```python
from build123d import *

# Parameters (mm, degrees)
SKETCH010_W     = 150
SKETCH010_H     = 108.5
PAD004_DEPTH    = 3
SKETCH011_W     = 3
SKETCH011_H     = 108.5
PAD005_DEPTH    = 36.8
SKETCH014_R     = 1.7
POCKET006_DEPTH = 5
SKETCH015_R     = 1.7
POCKET007_DEPTH = 5
POCKET010_DEPTH = 5
FILLET_R        = 2


with BuildPart() as part:
    # Sketch010 → Pad004 (new body)
    with BuildSketch(Plane.XY):
        with Locations((100.092897, -83.705943)):
            Rectangle(SKETCH010_W, SKETCH010_H)
    extrude(amount=PAD004_DEPTH)

    # Sketch011 (on Face5 of Pad004) → Pad005 (join)
    with BuildSketch(Plane(origin=(0, 0, 0), x_dir=(1, 0, 0), z_dir=(0, 0, -1))):
        with Locations((173.592904, 83.705948)):
            Rectangle(SKETCH011_W, SKETCH011_H)
        with Locations((26.592904, 83.705948)):
            Rectangle(SKETCH011_W, SKETCH011_H)
    extrude(amount=PAD005_DEPTH)

    # Sketch014 (on Face15 of Pad005) → Pocket006 (cut)
    with BuildSketch(Plane.YZ.offset(175.092904)):
        with Locations((-134.353821, -32.656531)):
            Circle(SKETCH014_R)
        with Locations((-33.353821, -32.656531)):
            Circle(SKETCH014_R)
    extrude(amount=-POCKET006_DEPTH, mode=Mode.SUBTRACT)

    # Sketch015 (on Face13 of Pocket006) → Pocket007 (cut)
    with BuildSketch(Plane(origin=(25.092904, 0, 0), x_dir=(0, -1, 0), z_dir=(-1, 0, 0))):
        with Locations((33.054447, -32.772871)):
            Circle(SKETCH015_R)
        with Locations((134.054447, -32.772871)):
            Circle(SKETCH015_R)
    extrude(amount=-POCKET007_DEPTH, mode=Mode.SUBTRACT)

    # Sketch018 (on Face13 of Pocket007) → Pocket010 (cut)
    with BuildSketch(Plane(origin=(25.092904, 0, 0), x_dir=(0, -1, 0), z_dir=(-1, 0, 0))):
        with BuildLine():
            ThreePointArc((48.372218, -10.337513), (46.972218, -8.937513), (45.572218, -10.337513))
            Line((45.572218, -10.337513), (45.572218, -26.337513))
            ThreePointArc((45.572218, -26.337513), (46.972218, -27.737513), (48.372218, -26.337513))
            Line((48.372218, -10.337513), (48.372218, -26.337513))
        make_face()
        with BuildLine():
            ThreePointArc((52.872218, -10.337513), (51.472218, -8.937513), (50.072218, -10.337513))
            Line((50.072218, -10.337513), (50.072218, -26.337513))
            ThreePointArc((50.072218, -26.337513), (51.472218, -27.737513), (52.872218, -26.337513))
            Line((52.872218, -10.337513), (52.872218, -26.337513))
        make_face()
        with BuildLine():
            ThreePointArc((57.372218, -10.337513), (55.972218, -8.937513), (54.572218, -10.337513))
            Line((54.572218, -10.337513), (54.572218, -26.337513))
            ThreePointArc((54.572218, -26.337513), (55.972218, -27.737513), (57.372218, -26.337513))
            Line((57.372218, -10.337513), (57.372218, -26.337513))
        make_face()
        with BuildLine():
            ThreePointArc((61.872218, -10.337513), (60.472218, -8.937513), (59.072218, -10.337513))
            Line((59.072218, -10.337513), (59.072218, -26.337513))
            ThreePointArc((59.072218, -26.337513), (60.472218, -27.737513), (61.872218, -26.337513))
            Line((61.872218, -10.337513), (61.872218, -26.337513))
        make_face()
        with BuildLine():
            ThreePointArc((66.372218, -10.337513), (64.972218, -8.937513), (63.572218, -10.337513))
            Line((63.572218, -10.337513), (63.572218, -26.337513))
            ThreePointArc((63.572218, -26.337513), (64.972218, -27.737513), (66.372218, -26.337513))
            Line((66.372218, -10.337513), (66.372218, -26.337513))
        make_face()
        with BuildLine():
            ThreePointArc((70.872218, -10.337513), (69.472218, -8.937513), (68.072218, -10.337513))
            Line((68.072218, -10.337513), (68.072218, -26.337513))
            ThreePointArc((68.072218, -26.337513), (69.472218, -27.737513), (70.872218, -26.337513))
            Line((70.872218, -10.337513), (70.872218, -26.337513))
        make_face()
    extrude(amount=-POCKET010_DEPTH, mode=Mode.SUBTRACT)

    # Fillet
    fillet_edges = [part.edges().sort_by_distance(p)[0] for p in [
        (25.092897, -83.705943, 3),
        (175.092897, -83.705943, 3),
    ]]
    fillet(fillet_edges, radius=FILLET_R)


solid = part.part
```
Geometry check sheet. Reference: the model listing, model coordinates, mm. A direction names the side the tool comes from. Round coordinates to 2 decimals unless told otherwise and drop trailing zeros. Loops run counter-clockwise (first coordinate to the right, second up) from the corner with the lowest first, then second, coordinate; pieces in that order, holes last. Notation, with made-up numbers: (58, 24) -> (73, 24) arc R10 ccw to (73, 34) -> close; hole circle Ø6 at (-20, 40). An arc over 180 degrees is marked (long way). Use a Markdown table: item, result.
(1) Go/stop test with a flat-tipped pin: P1, Ø10, axis at x = 120, y = -46.5, coming from the -Z side. Record where the tip stops, or that it passes through.
Calculated:
| item | result |
|---|---|
| P1 | z = 0 |
(2) Mould release check, pull along Y, two halves, no side actions. Record for faces 1 (the flat face through (99, -137.956, 1)), 2 (the flat face through (28.093, -83, -18)), 3 (the cylindrical face through (173.614, -34.703, -33.691)): released by +Y, released by -Y, zero draft, split by the parting line, or undercut.
Calculated:
| item | result |
|---|---|
| face 1 | released by -Y |
| face 2 | zero draft |
| face 3 | undercut |
(3) Sectioned sample at A-A (z = -17). Give the number of separate pieces and of enclosed holes in the cut face, then the cut area to 3 significant figures.
Calculated:
| item | result |
|---|---|
| separate pieces | 8 |
| enclosed holes | 0 |
| area | 601 mm² |
(4) Scan lines: probe 1 along X at (y, z) = (-108, -16.5); probe 2 along Z at (x, y) = (73, -108.5). Record each from-to range of solid material in increasing order.
Calculated:
| item | result |
|---|---|
| probe 1 | 25.09 to 28.09, 172.09 to 175.09 |
| probe 2 | 0 to 3 |
(5) Sectioned sample at C-C (x = 161.5). Enter the section's corners in (y, z), then the cut area to 4 significant figures.
Calculated:
| item | result |
|---|---|
| outline | (-137.96, 0) -> (-29.46, 0) -> (-29.46, 3) -> (-137.96, 3) -> close |
| area | 325.5 mm² |
(6) Set-up check for faces 4 (the cylindrical face through (173.614, -136.052, -32.582)), 5 (the flat face through (27, -84, -36.8)), 6 (the cylindrical face through (26.572, -34.625, -33.424)), 7 (the flat face through (172.093, -83, -18)), 8 (the flat face through (99, -29.456, 1)): record each of +Z, -Z, +X, -X, +Y, -Y from which the full face is reachable in a straight line by a thin tool's end or side.
Calculated:
| item | result |
|---|---|
| face 4 | +X |
| face 5 | -Z, +X, -X, +Y, -Y |
| face 6 | -X |
| face 7 | -Z, +Y, -Y |
| face 8 | +Z, -Z, +X, -X, +Y |
